```python
from build123d import *

# Parameters (mm, degrees)
SKETCH1_R           = 23.6982
SKETCH1_R_2         = 1.397
SKETCH1_R_3         = 4.0005
BOSS_EXTRUDE1_DEPTH = 3.175
SKETCH2_W           = 28.575
SKETCH2_H           = 57.15
BOSS_EXTRUDE2_DEPTH = 3.175
BOSS_EXTRUDE3_DEPTH = 3.175
SKETCH5_R           = 1.905
CUT_EXTRUDE2_DEPTH  = 6.35


with BuildPart() as part:
    # Sketch1 → Boss-Extrude1 (new body)
    with BuildSketch(Plane.ZY.offset(-268.497812887)):
        with Locations(Location((-22.229377206, 1.090549523, 0), (0, 0, 270))):
            Circle(SKETCH1_R)
        with Locations(Location((-4.785720318, -8.980550477, 0), (0, 0, 270))):
            Circle(SKETCH1_R_2, mode=Mode.SUBTRACT)
        with Locations(Location((-17.675988838, -1.538350477, 0), (0, 0, 270))):
            Circle(SKETCH1_R_2, mode=Mode.SUBTRACT)
        with Locations(Location((-26.782765574, -8.980550477, 0), (0, 0, 270))):
            Circle(SKETCH1_R_2, mode=Mode.SUBTRACT)
        with Locations(Location((-39.673034094, -1.538350477, 0), (0, 0, 270))):
            Circle(SKETCH1_R_2, mode=Mode.SUBTRACT)
        with Locations(Location((-28.674511466, 17.511649523, 0), (0, 0, 270))):
            Circle(SKETCH1_R_2, mode=Mode.SUBTRACT)
        with Locations(Location((-15.784242946, 10.069449523, 0), (0, 0, 270))):
            Circle(SKETCH1_R_2, mode=Mode.SUBTRACT)
        with Locations(Location((-11.230854578, -5.259450477, 0), (0, 0, 270))):
            Circle(SKETCH1_R_3, mode=Mode.SUBTRACT)
        with Locations(Location((-33.227899834, -5.259450477, 0), (0, 0, 270))):
            Circle(SKETCH1_R_3, mode=Mode.SUBTRACT)
        with Locations(Location((-22.229377206, 13.790549523, 0), (0, 0, 270))):
            Circle(SKETCH1_R_3, mode=Mode.SUBTRACT)
    extrude(amount=BOSS_EXTRUDE1_DEPTH)

    # Sketch2 → Boss-Extrude2 (add)
    with BuildSketch(Plane.XY.offset(-48.899377206)):
        with Locations((266.100312887, 9.853549523)):
            Rectangle(SKETCH2_W, SKETCH2_H)
    extrude(amount=BOSS_EXTRUDE2_DEPTH)

    # Sketch4 → Boss-Extrude3 (add)
    with BuildSketch(Plane(origin=(268.497812887, 0, 0), x_dir=(0, 0, -1), z_dir=(1, 0, 0))):
        with BuildLine():
            Line((45.724377206, -18.721450477), (45.724377206, -2.00616781))
            ThreePointArc((45.724377206, -2.00616781), (42.301350708, -11.507885419), (35.232812877, -18.721450477))
            Line((35.232812877, -18.721450477), (45.724377206, -18.721450477))
        make_face()
        with BuildLine():
            Line((45.724377206, 24.788749523), (22.229377206, 24.788749523))
            ThreePointArc((22.229377206, 24.788749523), (37.853366078, 18.908957279), (45.724377206, 4.187266856))
            Line((45.724377206, 4.187266856), (45.724377206, 24.788749523))
        make_face()
    extrude(amount=-BOSS_EXTRUDE3_DEPTH)

    # Sketch5 → Cut-Extrude2 (cut)
    with BuildSketch(Plane(origin=(0, 0, -48.899377206), x_dir=(-1, 0, 0), z_dir=(0, 0, -1))):
        with Locations((-274.875666904, -12.752450477)):
            Circle(SKETCH5_R)
        with Locations((-274.875666904, 29.538549523)):
            Circle(SKETCH5_R)
        with Locations((-255.825666904, 29.538549523)):
            Circle(SKETCH5_R)
        with Locations((-255.825666904, -12.752450477)):
            Circle(SKETCH5_R)
    extrude(amount=-CUT_EXTRUDE2_DEPTH, mode=Mode.SUBTRACT)


solid = part.part
```
Could you check a few things on this model? Use its own coordinates, in mm. A direction names the side the tool comes from. Coordinates: 2 decimals unless noted, no trailing zeros. Order: outer loops, then holes, each group sorted by start corner. A loop starts at its lowest first (then second) coordinate and runs counter-clockwise, first axis right, second up. Notation, with made-up numbers: M 13,25.5 L 29,25.5 A32 cw 29,54.5 Z; hole C 73.25,35.5 d10. An arc over 180 degrees is marked long. Use one line per item in the form item = value. Start each with the question number.
1. On a 3-axis mill with a long thin cutter (end or side, diameter ignored), from which of +Z, -Z, +X, -X, +Y, -Y can I reach the whole of each face in a straight line? I mean faces 1 (the cylindrical face through (273.06, 30.11, -47.33)), 2 (the flat face through (266, -18.721, -46)), 3 (the flat face through (268.498, 1, -22)). Say none if no direction works.
2. Suppose I cut it at C-C on z = -32.5. Write out the boundary of the cut face in (x, y), then the cut area to 3 significant figures.
3. For pin 1 (4 mm diameter, centred on y = 16, z = -30, fed in from +X); pin 2 (5 mm diameter, centred on x = 255.83, y = 29.54, fed in from +Z); pin 3 (1.6 mm diameter, centred on x = 267.5, z = -37, fed in from +Y), each with a flat end and sliding along its axis, tell me the tip position at first contact or that it passes through.
4. Suppose I cut it at A-A on y = 30.5. Write out the boundary of the cut face in (x, z), then the cut area to 3 significant figures.
5. We'd pull the mould along X, two halves only. Please class faces 4 (the flat face through (263, 10, -45.724)), 5 (the flat face through (265.323, 1, -22)), 6 (the cylindrical face through (257.73, 29.62, -47.33)): +X half, -X half, draft (parallel to the pull), parting line (faces both ways), or undercut.
6. Suppose I cut it at D-D on y = 20.5. Write out the boundary of the cut face in (x, z), then the cut area to 3 significant figures.
7. Please list where these lines run through material, in increasing order: line 1 (X direction, y = -14.5, z = -35.5); line 2 (Z direction, x = 259.75, y = 14.5); line 3 (Z direction, x = 267.25, y = -5).
8. Suppose I cut it at B-B on x = 267. Count the separate pieces of the cut face and the enclosed holes in it, then the cut area to 3 significant figures.
Geometry says:
q1.face_1 = +Z, -Z
q1.face_2 = -Z, +X, -X, -Y
q1.face_3 = +Z, +X, +Y, -Y
q2.outline = M 265.32,-20.27 L 268.5,-20.27 L 268.5,-9.19 L 265.32,-9.19 Z; M 265.32,-1.33 L 268.5,-1.33 L 268.5,24.79 L 265.32,24.79 Z
q2.area = 118 mm^2
q3.pin_1 = 268.5
q3.pin_2 = -45.72
q3.pin_3 = 24.79
q4.outline = M 251.81,-48.9 L 254.18,-48.9 L 254.18,-45.72 L 251.81,-45.72 Z; M 257.47,-48.9 L 273.23,-48.9 L 273.23,-45.72 L 257.47,-45.72 Z; M 276.52,-48.9 L 280.39,-48.9 L 280.39,-45.72 L 276.52,-45.72 Z
q4.area = 69.8 mm^2
q5.face_4 = draft
q5.face_5 = -X half
q5.face_6 = undercut
q6.outline = M 251.81,-48.9 L 280.39,-48.9 L 280.39,-45.72 L 268.5,-45.72 L 268.5,-8.63 L 265.32,-8.63 L 265.32,-45.72 L 251.81,-45.72 Z
q6.area = 208 mm^2
q7.line_1 = 265.32 to 268.5
q7.line_2 = -48.9 to -45.72
q7.line_3 = -48.9 to -37.22, -29.24 to -15.22, -7.24 to 0.67
q8.separate_pieces = 1
q8.enclosed_holes = 9
q8.area = 1,930 mm^2
